Verification items for this drawing (mm, ordinates from the low corner). A direction names the side the tool comes from. Coordinates: 2 decimals unless noted, no trailing zeros. Order: outer loops, then holes, each group sorted by start corner. A loop starts at its lowest first (then second) coordinate and runs counter-clockwise, first axis right, second up.
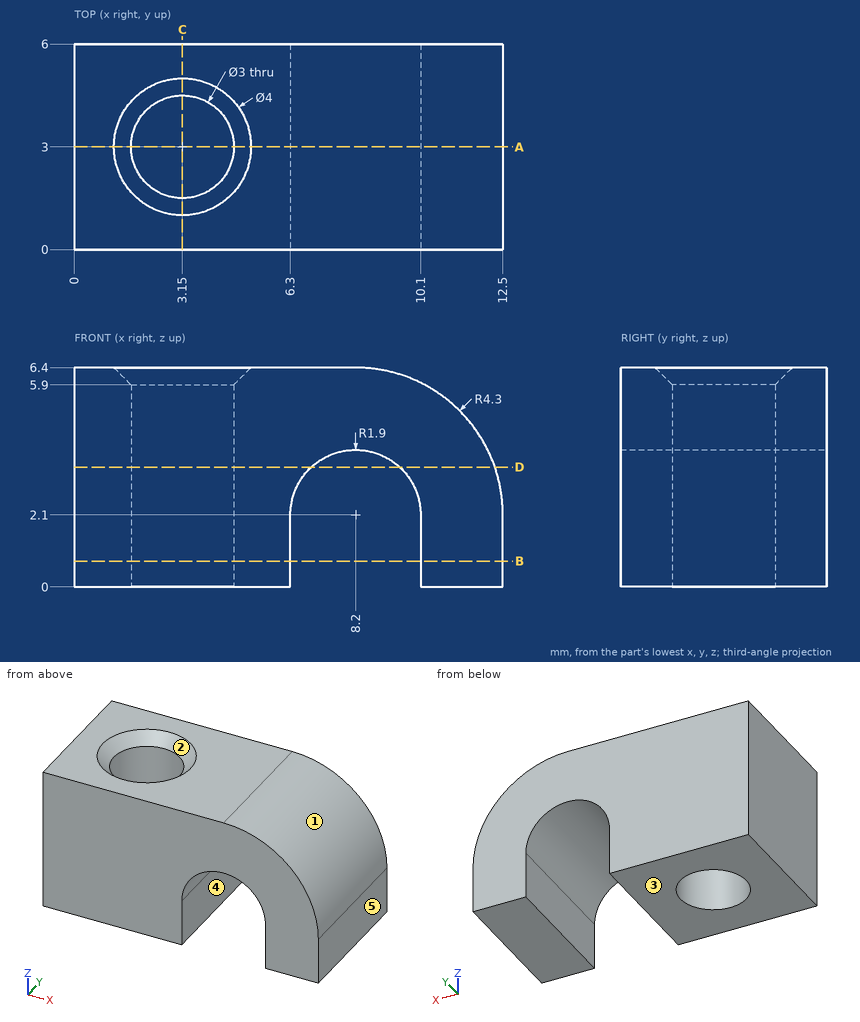
(1) Cross-section at B-B (z = 0.75). Enter the section's corners in (x, y), and give its area (3 significant figures).
Filled in:
outline: (0, 0) - (6.3, 0) - (6.3, 6) - (0, 6) - close; (10.1, 0) - (12.5, 0) - (12.5, 6) - (10.1, 6) - close; hole circle Ø3 at (3.15, 3)
area: 45.1 mm2
(2) Go/stop test with flat-tipped pins: P1, Ø1.8, axis at x = 3.15, y = 3, coming from the +Z side; P2, Ø3, axis at x = 8, y = 5.5, coming from the -Z side. Record where each tip stops, or that it passes through.
Filled in:
P1: passes through
P2: stops at z = 2.95
(3) Thickness scan on probe 1 along Y at (x, z) = (3.15, 4.3); probe 2 along X at (y, z) = (3.55, 0.75); probe 3 along X at (y, z) = (1.7, 3). Record the ranges inside material, lowest first.
Filled in:
probe 1: y = 0 to 1.5, 4.5 to 6
probe 2: x = 0 to 1.75, 4.55 to 6.3, 10.1 to 12.5
probe 3: x = 0 to 2.4, 3.9 to 6.53, 9.87 to 12.4
(4) Release check for a two-part mould opening along X. For the marked faces 1, 2 and 3 record: +X half, -X half, draft (parallel to the pull), parting line (faces both ways), or undercut.
Filled in:
face 1: +X half
face 2: undercut
face 3: draft
(5) Cross-section at C-C (x = 3.15). Enter the section's corners in (y, z).
Filled in:
outline: (0, 0) - (1.5, 0) - (1.5, 5.9) - (1, 6.4) - (0, 6.4) - close; (4.5, 0) - (6, 0) - (6, 6.4) - (5, 6.4) - (4.5, 5.9) - close
(6) Cross-section at A-A (y = 3). Enter the section's corners in (x, z), and give its area (3 significant figures).
Filled in:
outline: (0, 0) - (1.65, 0) - (1.65, 5.9) - (1.15, 6.4) - (0, 6.4) - close; (4.65, 0) - (6.3, 0) - (6.3, 2.1) arc R1.9 cw to (10.1, 2.1) - (10.1, 0) - (12.5, 0) - (12.5, 2.1) arc R4.3 ccw to (8.2, 6.4) - (5.15, 6.4) - (4.65, 5.9) - close
area: 42.9 mm2
(7) Tool access check on the marked faces 4 and 5. Record the directions out of +Z, -Z, +X, -X, +Y, -Y that give a thin tool (end or side, any length) a straight path to the whole face; none if there is none.
Filled in:
face 4: -Z, +Y, -Y
face 5: +Z, -Z, +X, +Y, -Y
(8) Cross-section at D-D (z = 3.5). Enter the section's corners in (x, y), and give its area (3 significant figures).
Filled in:
outline: (0, 0) - (6.92, 0) - (6.92, 6) - (0, 6) - close; (9.48, 0) - (12.27, 0) - (12.27, 6) - (9.48, 6) - close; hole circle Ø3 at (3.15, 3)
area: 51.1 mm2
